Source: CAD feature listing. Evaluate the final solid. Frame: model axes, mm. A direction names the side the tool comes from. Round coordinates to 2 decimals unless told otherwise and drop trailing zeros. Loops run counter-clockwise (first coordinate to the right, second up) from the corner with the lowest first, then second, coordinate; pieces in that order, holes last. Notation, with made-up numbers: (-11, 19) - (45, 19) arc R20 cw to (45, 51) - close; hole circle Ø1 at (70, 24). An arc over 180 degrees is marked (long way). Write item = value, one per line. Start each with the question number.
from build123d import *

# Parameters (mm, degrees)
F1_DEPTH = 10
F2_T     = -1
F3_DEPTH = 1.4
F4_W     = 3
F4_H     = 5
F4_W_2   = 3.991
F4_H_2   = 7.333
F5_DEPTH = 12


with BuildPart() as f1:
    # F0 (on Top) → F1 (new body)
    with BuildSketch(Plane.XY):
        with BuildLine():
            Line((-44.662655282, 31.9538097456), (-44.662655282, 21.9538097456))
            Line((-44.662655282, 21.9538097456), (-69.362655282, 21.9538097456))
            Line((-69.362655282, 21.9538097456), (-69.362655282, 1.9538097456))
            Line((-69.362655282, 1.9538097456), (-44.662655282, 1.9538097456))
            Line((-44.662655282, 1.9538097456), (-44.662655282, -8.0461902544))
            Line((-44.662655282, -8.0461902544), (-28.662655282, -8.0461902544))
            ThreePointArc((-28.662655282, -8.0461902544), (-24.662655282, -4.0461902544), (-20.662655282, -8.0461902544))
            Line((-20.662655282, -8.0461902544), (-4.662655282, -8.0461902544))
            Line((-4.662655282, -8.0461902544), (-4.662655282, 1.9538097456))
            Line((-4.662655282, 1.9538097456), (20.037344718, 1.9538097456))
            Line((20.037344718, 1.9538097456), (20.037344718, 21.9538097456))
            Line((20.037344718, 21.9538097456), (-4.662655282, 21.9538097456))
            Line((-4.662655282, 21.9538097456), (-4.662655282, 31.9538097456))
            Line((-4.662655282, 31.9538097456), (-44.662655282, 31.9538097456))
        make_face()
        with BuildLine():
            ThreePointArc((-20.662655282, -8.0461902544), (-24.662655282, -4.0461902544), (-28.662655282, -8.0461902544))
            Line((-28.662655282, -8.0461902544), (-20.662655282, -8.0461902544))
        make_face()
    extrude(amount=F1_DEPTH)

    # F2
    f2_openings = [f1.faces().sort_by_distance(p)[0] for p in [
        (-24.662655, 11.95381, 10),
    ]]
    offset(amount=F2_T, openings=f2_openings, kind=Kind.INTERSECTION)

    # F0 (on Top) → F3 (join)
    with BuildSketch(Plane.XY):
        with BuildLine():
            Line((-20.662655282, -8.0461902544), (-28.662655282, -8.0461902544))
            ThreePointArc((-28.662655282, -8.0461902544), (-24.662655282, -12.0461902544), (-20.662655282, -8.0461902544))
        make_face()
    extrude(amount=F3_DEPTH)

    # F4 (on face) → F5 (cut)
    with BuildSketch(Plane.XZ.offset(8.0461902544)):
        with Locations((-41.162655282, 5.5)):
            Rectangle(F4_W, F4_H)
        with Locations((-34.162655282, 5.5)):
            Rectangle(F4_W, F4_H)
        with Locations((-15.162655282, 5.5)):
            Rectangle(F4_W, F4_H)
        with Locations((-8.162655282, 5.5)):
            Rectangle(F4_W, F4_H)
        with Locations((0.837344718, 5.5)):
            Rectangle(F4_W, F4_H)
        with Locations((7.837344718, 5.5)):
            Rectangle(F4_W, F4_H)
        with Locations((14.837344718, 5.5)):
            Rectangle(F4_W, F4_H)
        with Locations((-24.658155282, 5.0665)):
            Rectangle(F4_W_2, F4_H_2)
    extrude(amount=-F5_DEPTH, mode=Mode.SUBTRACT)


solid = f1.part
(1) Access query for faces 1 (the face through (-57, 21.954, 5)), 2 (the face through (-43.663, -2, 5)), 3 (the face through (-25, -10, 1.4)). Directions: +Z, -Z, +X, -X, +Y, -Y. A direction counts if a zero-diameter tool reaches every point of the face in a straight line with its end or side. Return the directions, or none.
(2) Pin query (flat end, axial travel): P1, Ø5, axis at x = 6, z = 5.5, coming from the -Y side; P2, Ø0.5, axis at y = -7.5, z = 6, coming from the -X side; P3, Ø3, axis at x = -27, y = 5, coming from the +Z side; P4, Ø8, axis at x = 1.5, y = 17, coming from the -Z side. Return the tip coordinate at first contact, or that it passes through.
(3) Mould query, pull axis X, two halves, no side actions, for faces 4 (the face through (-4.663, 27, 5)), 5 (the face through (-5, 2, 10)), 6 (the face through (19.037, 12, 5)). Classes: +X half, -X half, draft (parallel to the pull), parting line (faces both ways), or undercut.
(4) Cut plane A-A (x = -8.5). Output: boundary loops of the cut face in (y, z).
(5) Cut plane D-D (z = 6). State how many separate pieces and enclosed holes the cut face has, and give its area (3 significant figures).
(6) Cut plane B-B (x = -61). Output: boundary loops of the cut face in (y, z).
(7) Material intervals for line 1 along Y through (x, z) = (-3, 3.25); line 2 along X through (y, z) = (22.5, 9.75); line 3 along X through (y, z) = (20, 7), sorted ascending. Write a range as from..to.
(8) Cut plane C-C (y = -4.5). Output: boundary loops of the cut face in (x, z), and give its area (3 significant figures).
Solution:
q1.face_1 = +Z, -Z, -X, +Y
q1.face_2 = +Z
q1.face_3 = -Y
q2.P1 = 1.95
q2.P2 = -44.66
q2.P3 = 1
q2.P4 = 0
q3.face_4 = +X half
q3.face_5 = draft
q3.face_6 = undercut
q4.outline = (-8.05, 0) - (31.95, 0) - (31.95, 10) - (30.95, 10) - (30.95, 1) - (-7.05, 1) - (-7.05, 3) - (-8.05, 3) - close; (-8.05, 8) - (-7.05, 8) - (-7.05, 10) - (-8.05, 10) - close
q5.separate_pieces = 8
q5.enclosed_holes = 0
q5.area = 230 mm^2
q6.outline = (1.95, 0) - (21.95, 0) - (21.95, 10) - (20.95, 10) - (20.95, 1) - (2.95, 1) - (2.95, 10) - (1.95, 10) - close
q7.line_1 = 1.95..2.95, 20.95..21.95
q7.line_2 = -44.66..-43.66, -5.66..-4.66
q7.line_3 = -69.36..-68.36, 19.04..20.04
q8.outline = (-44.66, 0) - (-4.66, 0) - (-4.66, 10) - (-5.66, 10) - (-5.66, 1) - (-43.66, 1) - (-43.66, 10) - (-44.66, 10) - close
q8.area = 58.0 mm^2
